CAD build for the part. Positions are in the model's coordinates, mm. Coordinates: 2 decimals unless noted, no trailing zeros. Order: outer loops, then holes, each group sorted by start corner. A loop starts at its lowest first (then second) coordinate and runs counter-clockwise, first axis right, second up. Notation, with made-up numbers: M 22,-14 L 49,-14 A9 cw 49,-9 Z; hole C -32,-14 d3. An arc over 180 degrees is marked long. Write item = value, one per line.
from build123d import *

# Parameters (mm, degrees)
SKETCH1_W           = 66.321579053
SKETCH1_H           = 6.35
BOSS_EXTRUDE2_DEPTH = 63.5
SKETCH2_W           = 19.05
SKETCH2_H           = 6.35
CUT_EXTRUDE1_DEPTH  = 25.4
SKETCH3_R           = 1.5875
CUT_EXTRUDE2_DEPTH  = 12.7
CUT_EXTRUDE3_START  = -12.7
SKETCH4_R           = 1.5875
CUT_EXTRUDE3_DEPTH  = 12.7
SKETCH5_R           = 5.08
SKETCH5_R_2         = 1.5875
BOSS_EXTRUDE3_DEPTH = 3.175
BOSS_EXTRUDE4_START = 3.175
SKETCH6_R           = 5.08
SKETCH6_R_2         = 1.5875
BOSS_EXTRUDE4_DEPTH = 3.175
SKETCH7_W           = 12.7
SKETCH7_H           = 22.225
CUT_EXTRUDE4_DEPTH  = 6.35
CUT_EXTRUDE5_START  = -22.225
CUT_EXTRUDE5_DEPTH  = 22.225
CUT_EXTRUDE8_START  = -22.225
CUT_EXTRUDE8_DEPTH  = 22.225


# Read off the part's stored shape, not the designer's step: Cut-Extrude5, Cut-Extrude8
with BuildPart() as part:
    # Sketch1 → Boss-Extrude2 (new body)
    with BuildSketch(Plane.XY):
        with Locations((-33.160789527, 5.715)):
            Rectangle(SKETCH1_W, SKETCH1_H)
    extrude(amount=BOSS_EXTRUDE2_DEPTH)

    # Sketch2 → Cut-Extrude1 (cut)
    with BuildSketch(Plane(origin=(0, 0, 0), x_dir=(0, 0, -1), z_dir=(1, 0, 0))):
        with Locations((-31.75, 5.715)):
            Rectangle(SKETCH2_W, SKETCH2_H)
    extrude(amount=-CUT_EXTRUDE1_DEPTH, mode=Mode.SUBTRACT)

    # Sketch3 → Cut-Extrude2 (cut)
    with BuildSketch(Plane(origin=(0, 0, 41.275), x_dir=(-1, 0, 0), z_dir=(0, 0, -1))):
        with Locations((18.7325, 5.715)):
            Circle(SKETCH3_R)
    extrude(amount=-CUT_EXTRUDE2_DEPTH, mode=Mode.SUBTRACT)

    # Sketch4 → Cut-Extrude3 (cut)
    with BuildSketch(Plane.XY.offset(22.225).offset(CUT_EXTRUDE3_START)):
        with Locations(Location((-18.7325, 5.715, 0), (0, 0, 180))):
            Circle(SKETCH4_R)
    extrude(amount=CUT_EXTRUDE3_DEPTH, mode=Mode.SUBTRACT)

    # Sketch5 → Boss-Extrude3 (add)
    with BuildSketch(Plane.XY.offset(63.5)):
        with Locations(Location((-18.7325, 12.573, 0), (0, 0, 226.468847833))):
            Circle(SKETCH5_R)
        with Locations((-18.7325, 12.573)):
            Circle(SKETCH5_R_2, mode=Mode.SUBTRACT)
    extrude(amount=BOSS_EXTRUDE3_DEPTH)

    # Sketch6 → Boss-Extrude4 (add)
    with BuildSketch(Plane(origin=(0, 0, 0), x_dir=(-1, 0, 0), z_dir=(0, 0, -1)).offset(BOSS_EXTRUDE4_START)):
        with Locations(Location((18.7325, 12.573, 0), (0, 0, 313.531152167))):
            Circle(SKETCH6_R)
        with Locations(Location((18.7325, 12.573, 0), (0, 0, 180))):
            Circle(SKETCH6_R_2, mode=Mode.SUBTRACT)
    extrude(amount=-BOSS_EXTRUDE4_DEPTH)

    # Sketch7 → Cut-Extrude4 (cut)
    with BuildSketch(Plane(origin=(0, 8.89, 0), x_dir=(1, 0, 0), z_dir=(0, 1, 0))):
        with Locations((-6.35, -11.1125)):
            Rectangle(SKETCH7_W, SKETCH7_H)
        with Locations((-6.35, -52.3875)):
            Rectangle(SKETCH7_W, SKETCH7_H)
    extrude(amount=-CUT_EXTRUDE4_DEPTH, mode=Mode.SUBTRACT)

    # Cut-Extrude5 outline → Cut-Extrude5 (cut)
    with BuildSketch(Plane(origin=(0, 0, 41.275), x_dir=(-1, 0, 0), z_dir=(0, 0, -1)).offset(CUT_EXTRUDE5_START)):
        with BuildLine():
            Line((12.7, 2.54), (15.068097478, 2.54))
            ThreePointArc((15.068097478, 2.54), (13.357223916, 3.734563769), (12.7, 5.715))
            Line((12.7, 5.715), (12.7, 2.54))
        make_face()
        with BuildLine():
            Line((12.7, 8.89), (12.7, 5.715))
            ThreePointArc((12.7, 5.715), (13.357223916, 7.695436231), (15.068097478, 8.89))
            Line((15.068097478, 8.89), (12.7, 8.89))
        make_face()
    extrude(amount=CUT_EXTRUDE5_DEPTH, mode=Mode.SUBTRACT)

    # Cut-Extrude8 outline → Cut-Extrude8 (cut)
    with BuildSketch(Plane.XY.offset(22.225).offset(CUT_EXTRUDE8_START)):
        with BuildLine():
            Line((-12.7, 8.89), (-15.0749, 8.89))
            ThreePointArc((-15.0749, 8.89), (-13.359413065, 7.697471627), (-12.7, 5.715))
            Line((-12.7, 5.715), (-12.7, 8.89))
        make_face()
        with BuildLine():
            Line((-12.7, 2.54), (-12.7, 5.715))
            ThreePointArc((-12.7, 5.715), (-13.359413065, 3.732528373), (-15.0749, 2.54))
            Line((-15.0749, 2.54), (-12.7, 2.54))
        make_face()
    extrude(amount=CUT_EXTRUDE8_DEPTH, mode=Mode.SUBTRACT)


solid = part.part
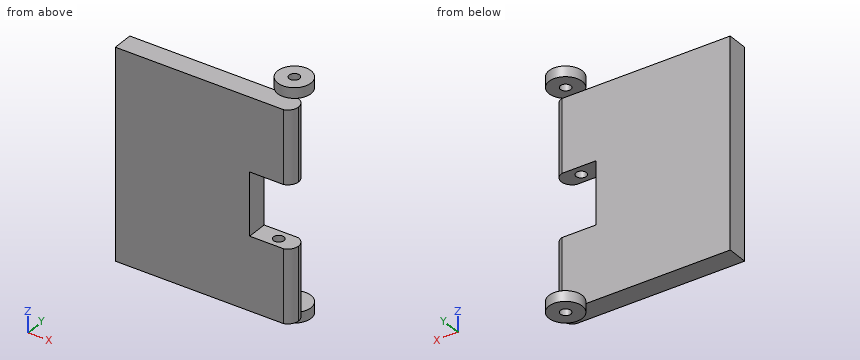
(1) Slice it at D-D, the plane z = 61.5. Write the cut outline in (x, y) (3 decimals).
Evaluation:
outline = M -66.322,2.54 L -15.068,2.54 A3.312 ccw -15.068,8.89 L -66.322,8.89 Z
(2) Slice it at B-B, the plane z = 51. Write the cut outline in (x, y) (1 decimal).
Evaluation:
outline = M -66.3,2.5 L -15.1,2.5 A3.3 ccw -15.1,8.9 L -66.3,8.9 Z; hole C -18.7,5.7 d3.2
(3) Pin check, flat tips, straight feed: pin 1 Ø6 at (y, z) = (14, 55) entering from -X; pin 2 Ø1.9 at (x, y) = (-34, 5.5) entering from +Z; pin 3 Ø3.5 at (x, y) = (-18.5, 5.5) entering from -Z; pin 4 Ø8 at (x, z) = (-39, 8) entering from +Y. Stop position of each tip, or through.
Evaluation:
pin_1 = through
pin_2 = 63.5
pin_3 = 0
pin_4 = 8.89
(4) Slice it at C-C, the plane x = -39.5. Write the cut outline in (y, z).
Evaluation:
outline = M 2.54,0 L 8.89,0 L 8.89,63.5 L 2.54,63.5 Z
(5) Slice it at A-A, the plane y = 16.25. Write the cut outline in (x, z) (3 decimals).
Evaluation:
outline = M -22.238,-3.175 L -15.227,-3.175 L -15.227,0 L -22.238,0 Z; M -22.238,63.5 L -15.227,63.5 L -15.227,66.675 L -22.238,66.675 Z
(6) Wall check: line 1 (Z direction, x = -20.5, y = 9.25) (3 decimals); line 2 (Y direction, x = -52, z = 20.5); line 3 (Z direction, x = -33, y = 5.75). Give the ranges that are in metal, low to high. Write a range as from..to.
Evaluation:
line_1 = -3.175..0, 63.5..66.675
line_2 = 2.54..8.89
line_3 = 0..63.5
